The listing builds one solid part. Answer for the finished solid, in the listing's coordinates (mm). Face numbers are marked on the shaded views. A direction names the side the tool comes from. Round coordinates to 2 decimals unless told otherwise and drop trailing zeros. Loops run counter-clockwise (first coordinate to the right, second up) from the corner with the lowest first, then second, coordinate; pieces in that order, holes last. Notation, with made-up numbers: (-1, 43) -> (42, 43) arc R8 cw to (42, 50) -> close; hole circle Ø8 at (-29, 73.25). An arc over 180 degrees is marked (long way). One line per question, with ' | ' between items.
Autodesk Inventor part; units mm, degrees
ref_plane "YZ Plane" through (0, 0, 0) normal (1, 0, 0) x (0, 1, 0)
ref_plane "XZ Plane" through (0, 0, 0) normal (0, 1, 0) x (-1, 0, 0)
ref_plane "XY Plane" through (0, 0, 0) normal (0, 0, 1) x (1, 0, 0)
sketch "Sketch1" plane through (0, 0, 0) normal (1, 0, 0) x (0, 1, 0)
  line L0 (0, 14.6) -> (6.55, 14.6)
  line L1 (6.55, 14.6) -> (6.55, 16.2)
  line L2 (0, 0) -> (0, 21.161) construction
  line L3 (6.55, 16.2) -> (0, 16.2)
  line L4 (0, 16.2) -> (0, 18.2)
  line L5 (0, 18.2) -> (8.5, 18.2)
  line L6 (8.5, 18.2) -> (8.5, 10.2659) construction
  line L7 (8.5, 13.1) -> (3, 13.1)
  line L8 (8.5, 18.2) -> (8.5, 13.1)
  line L9 (0, 2.5) -> (3, 2.5)
  line L10 (0, 0) -> (11.9587, 0) construction
  line L11 (3, 2.5) -> (3, 13.1)
  line L12 (0, 14.6) -> (0, 2.5)
  line L13 (6.55, 16.2) -> (8.5, 16.2)
  dimension "d0" = 6.55
  dimension "d1" = 14.6
  dimension "d2" = 16.2
  dimension "d3" = 2
  dimension "d4" = 8.5
  dimension "d5" = 1.5
  dimension "d6" = 3
  dimension "d7" = 2.5
revolve "Revolution1" add sketch "Sketch1" angle 360 about axis through (0, 0, 0) along (0, 1, 0) contours L3 L4 L5 L8 L13
sketch "Sketch5" plane through (0, 8.5, 0) normal (0, 1, 0) x (1, 0, 0)
  line L0 (0, 0) -> (0, 1)
  circle A0 centre (0, 1) radius 35
  circle A1 centre (0, 1) radius 36.5
  circle A2 centre (0, 0) radius 16.2
  dimension "d29" = 1
  dimension "d30" = 70
  dimension "d31" = 73
extrude "Extrusion2" add sketch "Sketch5" against normal blind 3 contours A0 | A2
extrude "Extrusion3" add sketch "Sketch5" against normal blind 23.7 contours A1
sketch "Sketch7" plane through (0, 5.5, 0) normal (0, -1, 0) x (1, 0, 0)
  circle A0 centre (0, 0) radius 16.2
extrude "Extrusion5" cut sketch "Sketch7" against normal blind 10
sketch "Sketch8" plane through (0, -15.2, 0) normal (0, -1, 0) x (1, 0, 0)
  circle A0 centre (0, -1) radius 36.5
  circle A1 centre (0, -1) radius 38
  point P0 (0, 0)
  dimension "d43" = 73
  dimension "d44" = 1
  dimension "d45" = 76
extrude "Extrusion6" add sketch "Sketch8" along normal blind 10 and the other way blind 5
sketch "Sketch10" plane through (0, 0, 0) normal (1, 0, 0) x (0, 1, 0)
  line L0 (-15.2, -1) -> (-15.2, -20.5)
  line L1 (-15.2, -36) -> (-15.2, 34)
  line L2 (-15.2, -20.5) -> (-15.2, -28)
  circle A0 centre (-15.2, -28) radius 9
  line L3 (-15.2, -19) -> (-25.2, -19)
  line L4 (-15.2, 35.5) -> (-15.2, -37.5)
  line L5 (-15.2, -37) -> (-25.2, -37)
  line L6 (-25.2, -37) -> (-25.2, -19)
  point P0 (0, 0)
  point P1 (-15.2, -1)
  point P2 (-25.2, -1)
  dimension "d60" = 19.5
  dimension "d61" = 7.5
  dimension "d62" = 18
extrude "Extrusion8" cut sketch "Sketch10" along normal through all
properties part number "Top of Housing.ipt v2"
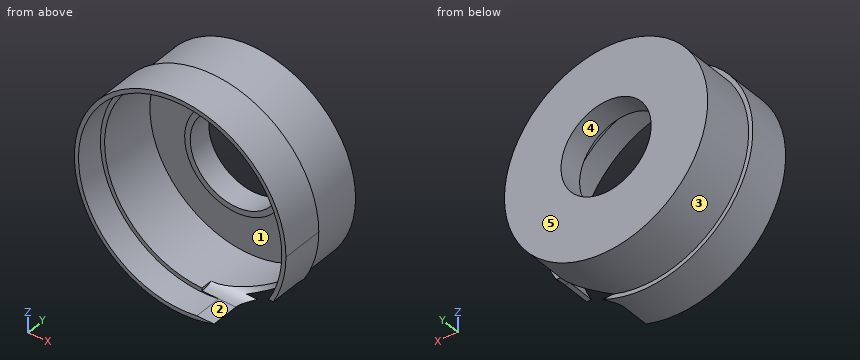
Q1. A cutting plane is placed at C-C on y = -19.5. Give the vertices of the cut face in (x, z).
Numbers:
outline: (6.02, -37) arc R36.5 cw (long way) to (31.75, -19) -> (33.47, -19) arc R38 ccw (long way) to (12.17, -37) -> close
Q2. Given pin 1 Ø1.9 at (x, y) = (32.5, -18.5) entering from -Z; pin 2 Ø22 at (x, z) = (-9.5, 7) entering from -Y; pin 3 Ø4 at (y, z) = (-5, -25.5) entering from -X, each flat-ended and moving along its own axis, determine where each tip first touches the part or whether it passes through.
Numbers:
pin 1: z = -19 | pin 2: y = 0 | pin 3: x = -28.74
Q3. Find the intervals of material crossed by line 1 (X direction, y = 4, z = 0); line 2 (X direction, y = -19.5, z = -1); line 3 (X direction, y = -9, z = -1), in increasing order. Write a range as from..to.
Numbers:
line 1: -36.49..-34.99, -18.2..-16.2, 16.2..18.2, 34.99..36.49 | line 2: -38..-36.5, 36.5..38 | line 3: -36.5..-35, 35..36.5
Q4. A cutting plane is placed at B-B on x = 7. Give the vertices of the cut face in (y, z), plus the area to 3 significant figures.
Numbers:
outline: (-25.2, -38.35) -> (-10.2, -38.35) -> (-10.2, -36.82) -> (8.5, -36.82) -> (8.5, -14.61) -> (0, -14.61) -> (0, -16.8) -> (5.5, -16.8) -> (5.5, -35.29) -> (-9.93, -35.29) arc R9 cw to (-15.2, -37) -> (-25.2, -37) -> close; (-25.2, 34.82) -> (-15.2, 34.82) -> (-15.2, 33.29) -> (5.5, 33.29) -> (5.5, 16.8) -> (0, 16.8) -> (0, 14.61) -> (8.5, 14.61) -> (8.5, 34.82) -> (-10.2, 34.82) -> (-10.2, 36.35) -> (-25.2, 36.35) -> close | area: 253 mm^2
Q5. For the marked faces 1 and 2, determine the directions among +Z, -Z, +X, -X, +Y, -Y from which every point of the face is accessible in a straight line to the end or side of a thin tool.
Numbers:
face 1: -Y | face 2: +X, -Y
Q6. A cutting plane is placed at D-D on y = -1. Give the vertices of the cut face in (x, z).
Numbers:
outline: circle Ø73 at (0, -1); hole circle Ø70 at (0, -1)
Q7. For a pull along X with two mould halves and no side action, classify the marked faces 3, 4 and 5 as pulls with the +X half, pulls with the -X half, needs draft (parallel to the pull), parting line crosses it, or undercut.
Numbers:
face 3: parting line crosses it | face 4: undercut | face 5: needs draft
Q8. A cutting plane is placed at A-A on z = 0. Give the vertices of the cut face in (x, y).
Numbers:
outline: (-37.99, -25.2) -> (-36.49, -25.2) -> (-36.49, -15.2) -> (-34.99, -15.2) -> (-34.99, 5.5) -> (-18.2, 5.5) -> (-18.2, 0) -> (-16.2, 0) -> (-16.2, 8.5) -> (-36.49, 8.5) -> (-36.49, -10.2) -> (-37.99, -10.2) -> close; (16.2, 0) -> (18.2, 0) -> (18.2, 5.5) -> (34.99, 5.5) -> (34.99, -15.2) -> (36.49, -15.2) -> (36.49, -25.2) -> (37.99, -25.2) -> (37.99, -10.2) -> (36.49, -10.2) -> (36.49, 8.5) -> (16.2, 8.5) -> close
